from build123d import *

# Parameters (mm, degrees)
BOSS_EXTRUDE1_DEPTH = 4.2
SKETCH2_R           = 1.1
CUT_EXTRUDE1_DEPTH  = 14.367834606
FILLET1_R           = 1
BOSS_EXTRUDE2_DEPTH = 0.8
BOSS_EXTRUDE3_DEPTH = 1
FILLET2_R           = 2


with BuildPart() as part:
    # Sketch1 → Boss-Extrude1 (new body)
    with BuildSketch(Plane.XY):
        with BuildLine():
            Line((0, -9), (0, -3.45))
            ThreePointArc((0, -3.45), (3.286405942, -1.049779017), (2, 2.811138559))
            Line((2, 2.811138559), (2, 6.5))
            Line((2, 6.5), (0.4, 6.5))
            Line((0.4, 6.5), (0.4, 1.393735986))
            ThreePointArc((0.4, 1.393735986), (0, -1.45), (-0.4, 1.393735986))
            Line((-0.4, 1.393735986), (-0.4, 6.5))
            Line((-0.4, 6.5), (-2, 6.5))
            Line((-2, 6.5), (-2, 2.811138559))
            ThreePointArc((-2, 2.811138559), (-3.45, 0), (-2, -2.811138559))
            Line((-2, -2.811138559), (-2, -9))
            Line((-2, -9), (-1.329280162, -10.84278761))
            ThreePointArc((-1.329280162, -10.84278761), (-0.124864136, -11.404416026), (0.436764281, -10.2))
            Line((0.436764281, -10.2), (0, -9))
        make_face()
    extrude(amount=BOSS_EXTRUDE1_DEPTH)

    # Sketch2 → Cut-Extrude1 (cut, through all)
    with BuildSketch(Plane.ZY.offset(2)):
        with Locations(Location((2.1, 4.65556928, 0), (0, 0, 270))):
            Circle(SKETCH2_R)
    extrude(amount=-CUT_EXTRUDE1_DEPTH, mode=Mode.SUBTRACT)

    # Fillet1
    fillet1_edges = [part.edges().sort_by_distance(p)[0] for p in [
        (-1.2, 6.5, 0),
        (1.2, 6.5, 0),
        (1.2, 6.5, 4.2),
        (-1.2, 6.5, 4.2),
    ]]
    fillet(fillet1_edges, radius=FILLET1_R)

    # Sketch3 → Boss-Extrude2 (add)
    with BuildSketch(Plane.XY.offset(4.2)):
        with BuildLine():
            Line((-1.45, 0), (-3.45, 0))
            ThreePointArc((-3.45, 0), (-3.066145789, -1.581534065), (-2, -2.811138559))
            Line((-2, -2.811138559), (-2, -9))
            Line((-2, -9), (-1.329280162, -10.84278761))
            ThreePointArc((-1.329280162, -10.84278761), (-0.124864136, -11.404416026), (0.436764281, -10.2))
            Line((0.436764281, -10.2), (0, -9))
            Line((0, -9), (0, -3.45))
            ThreePointArc((0, -3.45), (2.439518395, -2.439518395), (3.45, 0))
            Line((3.45, 0), (1.45, 0))
            ThreePointArc((1.45, 0), (0, -1.45), (-1.45, 0))
        make_face()
    extrude(amount=BOSS_EXTRUDE2_DEPTH)

    # Sketch4 → Boss-Extrude3 (add)
    with BuildSketch(Plane.XY.offset(5)):
        with BuildLine():
            ThreePointArc((1.45, 0), (1.158123482, 0.872496418), (0.4, 1.393735986))
            ThreePointArc((0.4, 1.393735986), (-0.872496418, 1.158123482), (-1.45, 0))
            ThreePointArc((-1.45, 0), (0, -1.45), (1.45, 0))
        make_face()
        with BuildLine():
            ThreePointArc((3.45, 0), (3.066145789, 1.581534065), (2, 2.811138559))
            ThreePointArc((2, 2.811138559), (-1.581534065, 3.066145789), (-3.45, 0))
            Line((-3.45, 0), (-1.45, 0))
            ThreePointArc((-1.45, 0), (-0.872496418, 1.158123482), (0.4, 1.393735986))
            ThreePointArc((0.4, 1.393735986), (1.158123482, 0.872496418), (1.45, 0))
            Line((1.45, 0), (3.45, 0))
        make_face()
        with BuildLine():
            ThreePointArc((0, -3.45), (2.439518395, -2.439518395), (3.45, 0))
            Line((3.45, 0), (1.45, 0))
            ThreePointArc((1.45, 0), (0, -1.45), (-1.45, 0))
            Line((-1.45, 0), (-3.45, 0))
            ThreePointArc((-3.45, 0), (-3.066145789, -1.581534065), (-2, -2.811138559))
            Line((-2, -2.811138559), (-2, -9))
            Line((-2, -9), (-1.329280162, -10.84278761))
            ThreePointArc((-1.329280162, -10.84278761), (-0.124864136, -11.404416026), (0.436764281, -10.2))
            Line((0.436764281, -10.2), (0, -9))
            Line((0, -9), (0, -3.45))
        make_face()
    extrude(amount=BOSS_EXTRUDE3_DEPTH)

    # Fillet2
    fillet2_edges = [part.edges().sort_by_distance(p)[0] for p in [
        (0, -3.45, 3),
        (0, -9, 3),
        (-2, -9, 3),
        (-2, -2.811138559, 3),
    ]]
    fillet(fillet2_edges, radius=FILLET2_R)


solid = part.part
Input: part model. Units: mm. Frame: model coordinates. A direction names the side the tool comes from. Coordinates: 2 decimals unless noted, no trailing zeros. Order: outer loops, then holes, each group sorted by start corner. A loop starts at its lowest first (then second) coordinate and runs counter-clockwise, first axis right, second up.
1. Draft query along X for faces 6 (the flat face through (-0.4, 3, 2)), 7 (the flat face through (0, 1, 5)), 8 (the cylindrical face through (-1.211, 6.199, 3.915)), 9 (the flat face through (-1.6, -10.1, 3)). Return one class per face: +X half, -X half, draft (parallel to the pull), parting line (faces both ways), or undercut.
Checked values:
face 6: undercut
face 7: undercut
face 8: draft
face 9: -X half
2. Ray query, line 1 along X through (y, z) = (0, 3); line 2 along Y through (x, z) = (1.25, 3.05); line 3 along Z through (x, y) = (1.25, 1). Return the intervals inside material, ascending.
Checked values:
line 1: x = -3.45 to -1.45, 1.45 to 3.45
line 2: y = -3.22 to -0.73, 0.73 to 4.1, 5.21 to 6.5
line 3: z = 0 to 4.2, 5 to 6
3. Cut plane A-A, the plane z = 2.1. Return loops of the section in (x, y), plus the area to 3 significant figures.
Checked values:
outline: (-2.53, -2.34) arc R2 cw to (-2, -3.7) - (-2, -8.65) arc R2 ccw to (-1.88, -9.33) - (-1.33, -10.84) arc R0.94 ccw to (0.44, -10.2) - (0.12, -9.33) arc R2 cw to (0, -8.65) - (0, -5.07) arc R2 cw to (1.27, -3.21) arc R3.45 ccw to (2, 2.81) - (2, 3.56) - (0.4, 3.56) - (0.4, 1.39) arc R1.45 cw (long way) to (-0.4, 1.39) - (-0.4, 3.56) - (-2, 3.56) - (-2, 2.81) arc R3.45 ccw to start; (-2, 5.76) - (-0.4, 5.76) - (-0.4, 6.5) - (-2, 6.5) - close; (0.4, 5.76) - (2, 5.76) - (2, 6.5) - (0.4, 6.5) - close
area: 49.2 mm2
4. Contact query for flat-ended pins moving along their axis: P1, Ø1.3, axis at y = 3.5, z = 3, coming from the -X side; P2, Ø3.5, axis at y = 4.66, z = 2.1, coming from the +X side; P3, Ø3, axis at y = 4, z = 3, coming from the +X side; P4, Ø1.8, axis at y = 4.66, z = 2.1, coming from the +X side. Output: stop coordinate, or through.
Checked values:
P1: stops at x = -2
P2: stops at x = 2
P3: stops at x = 2.38
P4: passes through
5. Cut plane B-B, the plane x = -0.75. Return loops of the section in (y, z), plus the area to 3 significant figures.
Checked values:
outline: (-11.41, 0) - (-1.24, 0) - (-1.24, 5) - (3.37, 5) - (3.37, 6) - (-11.41, 6) - close; (1.24, 0) - (5.5, 0) arc R1 ccw to (6.5, 1) - (6.5, 3.2) arc R1 ccw to (5.5, 4.2) - (1.24, 4.2) - close; hole circle Ø2.2 at (4.66, 2.1)
area: 83.5 mm2
6. Cut plane C-C, the plane z = 1.2. Return loops of the section in (x, y), plus the area to 3 significant figures.
Checked values:
outline: (-2.53, -2.34) arc R2 cw to (-2, -3.7) - (-2, -8.65) arc R2 ccw to (-1.88, -9.33) - (-1.33, -10.84) arc R0.94 ccw to (0.44, -10.2) - (0.12, -9.33) arc R2 cw to (0, -8.65) - (0, -5.07) arc R2 cw to (1.27, -3.21) arc R3.45 ccw to (2, 2.81) - (2, 4.02) - (0.4, 4.02) - (0.4, 1.39) arc R1.45 cw (long way) to (-0.4, 1.39) - (-0.4, 4.02) - (-2, 4.02) - (-2, 2.81) arc R3.45 ccw to start; (-2, 5.29) - (-0.4, 5.29) - (-0.4, 6.5) - (-2, 6.5) - close; (0.4, 5.29) - (2, 5.29) - (2, 6.5) - (0.4, 6.5) - close
area: 52.2 mm2
7. Access query for faces 1 (the flat face through (-2, 3, 2)), 2 (the flat face through (0.28, -9.77, 2.96)), 3 (the flat face through (-2, -6, 3)), 4 (the flat face through (0.4, 3, 2)), 5 (the flat face through (-1.6, 2.8, 4.2)). Directions: +Z, -Z, +X, -X, +Y, -Y. A direction counts if a zero-diameter tool reaches every point of the face in a straight line with its end or side. Return the directions, or none.
Checked values:
face 1: +Z, -Z, -X, +Y
face 2: +Z, -Z, +X
face 3: +Z, -Z, -X, -Y
face 4: -Z, +Y
face 5: +X, -X, +Y
8. Cut plane D-D, the plane x = 3. Return loops of the section in (y, z), plus the area to 3 significant figures.
Checked values:
outline: (-1.7, 0) - (1.7, 0) - (1.7, 4.2) - (0, 4.2) - (0, 5) - (1.7, 5) - (1.7, 6) - (-1.7, 6) - close
area: 19.1 mm2
